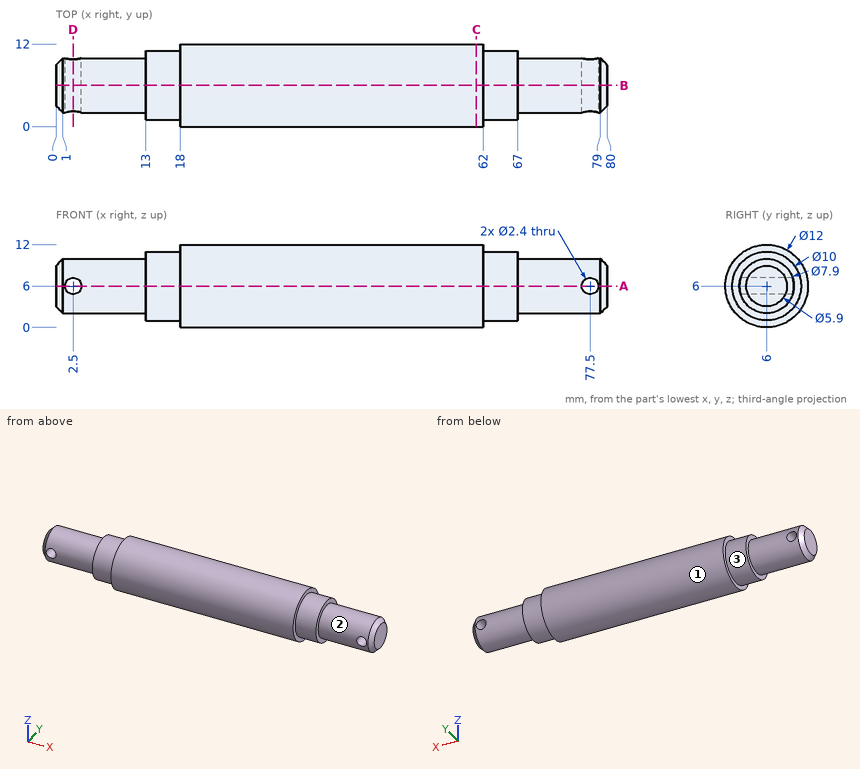
Job drawing, mm, ordinate dimensions from the low corner. One solid piece. A direction names the side the tool comes from. Coordinates: 2 decimals unless noted, no trailing zeros. Write each loop counter-clockwise with the first axis right and the second up, starting at its lowest first coordinate (ties: lowest second). Pieces come first, ordered by that corner, then holes.
Item 1: Slice it at A-A (z = 6). Count the separate pieces of the cut face and the enclosed holes in it, and give its area (3 significant figures).
Item 2: Slice it at D-D (x = 2.5). Write the cut outline in (y, z), and give its area (3 significant figures).
Item 3: Which spindle directions (+Z, -Z, +X, -X, +Y, -Y) get a long thin tool onto all of the face, cutting with end or side? Do the marked faces 1, 2 and 3. Say none if no direction does.
Item 4: Slice it at B-B (y = 6). Write the cut outline in (x, z), and give its area (3 significant figures).
Item 5: Pin check, flat tips, straight feed: pin 1 (4 mm diameter, centred on x = 65.5, y = 10, fed in from -Z); pin 2 (4 mm diameter, centred on x = 2.5, z = 6, fed in from -Y); pin 3 (5 mm diameter, centred on x = 26.5, z = 2.5, fed in from +Y); pin 4 (1.5 mm diameter, centred on y = 5.5, z = 3, fed in from +X). Stop position of each tip, or through.
Item 6: Probe line 1 (X direction, y = 7.75, z = 6); line 2 (X direction, y = 3.75, z = 6.5); line 3 (Z direction, x = 2.5, y = 7). List the from-to ranges inside material, lowest first.
Item 7: Slice it at C-C (x = 61). Write the cut outline in (y, z), and give its area (3 significant figures).
Results found:
1. separate pieces: 3
1. enclosed holes: 0
1. area: 793 mm2
2. outline: (2.24, 4.8) arc R3.95 ccw to (9.76, 4.8) - close; (2.24, 7.2) - (9.76, 7.2) arc R3.95 ccw to start
2. area: 30.4 mm2
3. face 1: +X, -X
3. face 2: +X
3. face 3: -X
4. outline: (0, 3.05) - (1, 2.05) - (13, 2.05) - (13, 1) - (18, 1) - (18, 0) - (62, 0) - (62, 1) - (67, 1) - (67, 2.05) - (79, 2.05) - (80, 3.05) - (80, 8.95) - (79, 9.95) - (67, 9.95) - (67, 11) - (62, 11) - (62, 12) - (18, 12) - (18, 11) - (13, 11) - (13, 9.95) - (1, 9.95) - (0, 8.95) - close; hole circle Ø2.4 at (2.5, 6); hole circle Ø2.4 at (77.5, 6)
4. area: 822 mm2
5. pin 1: stops at z = 1.42
5. pin 2: stops at y = 2.05
5. pin 3: stops at y = 11.92
5. pin 4: stops at x = 80
6. line 1: x = 0 to 1.3, 3.7 to 76.3, 78.7 to 80
6. line 2: x = 0 to 1.41, 3.59 to 76.41, 78.59 to 80
6. line 3: z = 2.18 to 4.8, 7.2 to 9.82
7. outline: circle Ø12 at (6, 6)
7. area: 113 mm2
